Verification items for the finished model (mm, model axes). Round coordinates to 2 decimals unless told otherwise and drop trailing zeros. Write each loop counter-clockwise with the first axis right and the second up, starting at its lowest first coordinate (ties: lowest second). Pieces come first, ordered by that corner, then holes. Notation, with made-up numbers: M -29.5,1 L 26.5,1 A24 ccw 26.5,11 Z; hole C 81,40.25 d10. An arc over 180 degrees is marked long. Write each question's results on one line, items separated by ' | '.
from build123d import *

# Parameters (mm, degrees)
SKETCH1_R           = 6.35
BOSS_EXTRUDE1_DEPTH = 831.85
BOSS_EXTRUDE2_START = 25.4
BOSS_EXTRUDE2_DEPTH = 11.049


with BuildPart() as part:
    # Sketch1 → Boss-Extrude1 (new body)
    with BuildSketch(Plane(origin=(0, 0, 0), x_dir=(1, 0, 0), z_dir=(0, 1, 0))):
        Circle(SKETCH1_R)
    extrude(amount=BOSS_EXTRUDE1_DEPTH)

    # Sketch3 → Boss-Extrude2 (add)
    with BuildSketch(Plane(origin=(0, 0, 0), x_dir=(1, 0, 0), z_dir=(0, 1, 0)).offset(BOSS_EXTRUDE2_START)):
        Polygon((9.876865428, 4.838907863), (0.747815578, 10.973070302), (-9.129049851, 6.134162439), (-9.876865428, -4.838907863), (-0.747815578, -10.973070302), (9.129049851, -6.134162439), align=None)
    extrude(amount=BOSS_EXTRUDE2_DEPTH)


solid = part.part
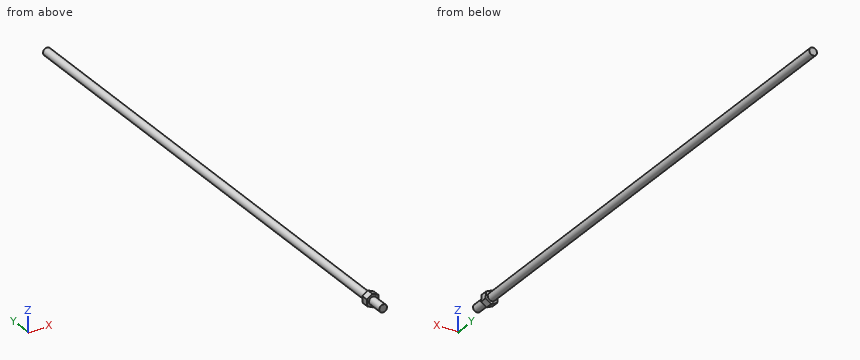
1) Material ranges on line 1 (Z direction, x = 1.5, y = 339.5); line 2 (X direction, y = 77, z = -4), recorded low to high. Write a range as [from, to].
Calculated:
line 1: z = [-6.17, 6.17] | line 2: x = [-4.93, 4.93]
2) Sectioned sample at A-A, the plane z = 0. Record the cut outline in (x, y), and give its area (3 significant figures).
Calculated:
outline: M -9.55,25.4 L -6.35,25.4 L -6.35,0 L 6.35,0 L 6.35,25.4 L 9.55,25.4 L 9.55,36.45 L 6.35,36.45 L 6.35,831.85 L -6.35,831.85 L -6.35,36.45 L -9.55,36.45 Z | area: 10,600 mm²
3) Depth check by flat-ended pin: P1, Ø2, axis at x = 6, z = -4.5, coming from the +Y side; P2, Ø2, axis at x = 1.5, y = 742.5, coming from the +Z side; P3, Ø10, axis at y = 656, z = 4.5, coming from the -X side; P4, Ø1.5, axis at y = 683, z = -7.5, coming from the -X side. Enter the tip coordinate at first touch or a pass-through.
Calculated:
P1: stops at y = 36.45 | P2: stops at z = 6.33 | P3: stops at x = -6.35 | P4: passes through
4) Sectioned sample at B-B, the plane y = 474. Record the cut outline in (x, z).
Calculated:
outline: C 0,0 d12.7
